Design review of the part built by this model. Coordinates are the model's own, in mm. A direction names the side the tool comes from. Coordinates: 2 decimals unless noted, no trailing zeros. Loops run counter-clockwise (first coordinate to the right, second up) from the corner with the lowest first, then second, coordinate; pieces in that order, holes last. Notation, with made-up numbers: (25.5, 80) - (76.5, 80) arc R19 cw to (76.5, 91) - close; hole circle Ø8 at (-23.5, 18.25). An arc over 180 degrees is marked (long way). Use one line per item in the form item = value. Start each with the question number.
(1) Clearance check with flat-ended pins moving along their axes: pin 1 Ø1.5 at (y, z) = (98.5, -0.5) entering from +X; pin 2 Ø1 at (x, z) = (0.5, 1) entering from +Y; pin 3 Ø0.9 at (x, z) = (-4.5, 0.5) entering from +Y. State where each tip first meets the part, or that it passes through.
(2) Tool access review of faces 1 (the face through (-5, 75, -1.5)), 2 (the face through (2, 3, 0)): name each direction out of +Z, -Z, +X, -X, +Y, -Y from which nothing blocks a thin tool from reaching the whole face with its end or side.
(3) Add section A-A (z = 0.05). State the section outline as (x, y) points, plus the area to 3 significant figures.
(4) The part is to be moulded in two halves that separate along X. For faces 3 (the face through (-7.5, 80, 0)), 4 (the face through (7.5, 1, 0)), 5 (the face through (-5, 161, 0)), say which applies: pulls with the +X half, pulls with the -X half, needs draft (parallel to the pull), parting line crosses it, or undercut.
(5) For L1, parallel to Y at x = 0.25, z = -0.95; L2, parallel to Y at x = -3.75, z = -0.05; L3, parallel to X at y = 44, z = -0.4, list the stretches that pass through material, from the lowest coordinate up.
(6) Add section C-C (y = 52.5). State the section outline as (x, z) points.
(7) Add section B-B (x = -0.75). State the section outline as (y, z) points.
```python
from build123d import *

# Parameters (mm, degrees)
SKETCH1_W           = 15
SKETCH1_H           = 3
BOSS_EXTRUDE1_DEPTH = 3
SKETCH2_W           = 5
SKETCH2_H           = 3
BOSS_EXTRUDE2_DEPTH = 160
CUT_EXTRUDE1_DEPTH  = 2


with BuildPart() as part:
    # Sketch1 → Boss-Extrude1 (new body)
    with BuildSketch(Plane(origin=(0, 0, 0), x_dir=(1, 0, 0), z_dir=(0, 1, 0))):
        Rectangle(SKETCH1_W, SKETCH1_H)
    extrude(amount=BOSS_EXTRUDE1_DEPTH)

    # Sketch2 → Boss-Extrude2 (add)
    with BuildSketch(Plane(origin=(0, 3, 0), x_dir=(1, 0, 0), z_dir=(0, 1, 0))):
        with Locations((-5, 0)):
            Rectangle(SKETCH2_W, SKETCH2_H)
    extrude(amount=BOSS_EXTRUDE2_DEPTH)

    # Sketch3 → Cut-Extrude1 (cut)
    with BuildSketch(Plane(origin=(0, 163, 0), x_dir=(1, 0, 0), z_dir=(0, 1, 0))):
        Polygon((-6, 1), (-7.5, 1), (-7.5, -1), (-6, -1), (-6, -1.5), (-4, -1.5), (-4, -1), (-2.5, -1), (-2.5, 1), (-4, 1), (-4, 1.5), (-6, 1.5), align=None)
    extrude(amount=-CUT_EXTRUDE1_DEPTH, mode=Mode.SUBTRACT)


solid = part.part
```
Computed values:
q1.pin_1 = -2.5
q1.pin_2 = 3
q1.pin_3 = 161
q2.face_1 = -Z, +X, -X, +Y, -Y
q2.face_2 = +Z, -Z, +X, +Y
q3.outline = (-7.5, 0) - (7.5, 0) - (7.5, 3) - (-2.5, 3) - (-2.5, 161) - (-7.5, 161) - close
q3.area = 835 mm^2
q4.face_3 = pulls with the -X half
q4.face_4 = pulls with the +X half
q4.face_5 = undercut
q5.L1 = 0 to 3
q5.L2 = 0 to 161
q5.L3 = -7.5 to -2.5
q6.outline = (-7.5, -1.5) - (-2.5, -1.5) - (-2.5, 1.5) - (-7.5, 1.5) - close
q7.outline = (0, -1.5) - (3, -1.5) - (3, 1.5) - (0, 1.5) - close
